The listing builds one solid part. Answer for the finished solid, in the listing's coordinates (mm). A direction names the side the tool comes from. Coordinates: 2 decimals unless noted, no trailing zeros. Order: outer loops, then holes, each group sorted by start corner. A loop starts at its lowest first (then second) coordinate and runs counter-clockwise, first axis right, second up. Notation, with made-up numbers: (7.5, 21.5) -> (62.5, 21.5) arc R19 ccw to (62.5, 57.5) -> close; hole circle Ø2 at (-36, -27.5). An arc over 180 degrees is marked (long way). Write item = value, one per line.
from build123d import *

# Parameters (mm, degrees)
SKETCH_W     = 80.45
SKETCH_H     = 153.35
SKETCH_R     = 1.5
PAD_DEPTH    = 3
SKETCH001_W  = 60.3
SKETCH001_H  = 10
POCKET_DEPTH = 3.001


with BuildPart() as part:
    # Sketch → Pad (new body)
    with BuildSketch(Plane.XY):
        with Locations((40.225, 76.675)):
            Rectangle(SKETCH_W, SKETCH_H)
        with Locations((68.4, 9)):
            Circle(SKETCH_R, mode=Mode.SUBTRACT)
        with Locations((70.45, 144.35)):
            Circle(SKETCH_R, mode=Mode.SUBTRACT)
        with Locations((52.45, 144.35)):
            Circle(SKETCH_R, mode=Mode.SUBTRACT)
        with Locations((34.45, 144.35)):
            Circle(SKETCH_R, mode=Mode.SUBTRACT)
        with Locations((31, 91.35)):
            Circle(SKETCH_R, mode=Mode.SUBTRACT)
        with Locations((51, 91.35)):
            Circle(SKETCH_R, mode=Mode.SUBTRACT)
    extrude(amount=PAD_DEPTH)

    # Sketch001 → Pocket (cut, through all)
    with BuildSketch(Plane.XY.offset(3)):
        with Locations((30.15, 5)):
            Rectangle(SKETCH001_W, SKETCH001_H)
    extrude(amount=-POCKET_DEPTH, mode=Mode.SUBTRACT)


solid = part.part
Q1. Each of these flat-tipped pins is pushed along its axis until it touches: pin 1 Ø1.5 at (x, z) = (44, 1.5) entering from -Y; pin 2 Ø0.9 at (y, z) = (7, 1.5) entering from -X. Where does it stop, or does it pass through?
The answers:
pin_1 = 10
pin_2 = 60.3
Q2. Section B-B, the plane x = 34.45 is taken. Give the vertices of the cut face in (y, z), plus the area to 3 significant figures.
The answers:
outline = (10, 0) -> (142.85, 0) -> (142.85, 3) -> (10, 3) -> close; (145.85, 0) -> (153.35, 0) -> (153.35, 3) -> (145.85, 3) -> close
area = 421 mm2
Q3. Find the intervals of material crossed by line 1 along X through (y, z) = (144.35, 1.25); line 2 along Y through (x, z) = (31, 2.1); line 3 along Y through (x, z) = (70.45, 1.3), in increasing order.
The answers:
line_1 = 0 to 32.95, 35.95 to 50.95, 53.95 to 68.95, 71.95 to 80.45
line_2 = 10 to 89.85, 92.85 to 153.35
line_3 = 0 to 142.85, 145.85 to 153.35
Q4. Section C-C, the plane y = 91.35 is taken. Give the vertices of the cut face in (x, z).
The answers:
outline = (0, 0) -> (29.5, 0) -> (29.5, 3) -> (0, 3) -> close; (32.5, 0) -> (49.5, 0) -> (49.5, 3) -> (32.5, 3) -> close; (52.5, 0) -> (80.45, 0) -> (80.45, 3) -> (52.5, 3) -> close
Q5. The mould has two halves that part along Y. Classify faces 1 (the face through (60.3, 5, 2)), 2 (the face through (70, 0, 1)), 3 (the face through (34.255, 145.837, 1.479)), 4 (the face through (40, 153.35, 1)): released by +Y, released by -Y, zero draft, split by the parting line, or undercut.
The answers:
face_1 = zero draft
face_2 = released by -Y
face_3 = undercut
face_4 = released by +Y
Q6. A tool of negligible diameter and unlimited length cuts with its end or side. For faces 5 (the face through (66.9, 9.07, 1.48)), 6 (the face through (30, 10, 2)), from which of +Z, -Z, +X, -X, +Y, -Y can it reach the whole face along a straight path? Write none if from no direction.
The answers:
face_5 = +Z, -Z
face_6 = +Z, -Z, -X, -Y
Q7. Section D-D, the plane z = 0.45 is taken. Give the vertices of the cut face in (x, y).
The answers:
outline = (0, 10) -> (60.3, 10) -> (60.3, 0) -> (80.45, 0) -> (80.45, 153.35) -> (0, 153.35) -> close; hole circle Ø3 at (31, 91.35); hole circle Ø3 at (34.45, 144.35); hole circle Ø3 at (51, 91.35); hole circle Ø3 at (52.45, 144.35); hole circle Ø3 at (68.4, 9); hole circle Ø3 at (70.45, 144.35)
Q8. Section A-A, the plane y = 144.35 is taken. Give the vertices of the cut face in (x, z).
The answers:
outline = (0, 0) -> (32.95, 0) -> (32.95, 3) -> (0, 3) -> close; (35.95, 0) -> (50.95, 0) -> (50.95, 3) -> (35.95, 3) -> close; (53.95, 0) -> (68.95, 0) -> (68.95, 3) -> (53.95, 3) -> close; (71.95, 0) -> (80.45, 0) -> (80.45, 3) -> (71.95, 3) -> close
